Work out the finished part from the listing and answer in its coordinate system (mm). A direction names the side the tool comes from. Coordinates: 2 decimals unless noted, no trailing zeros. Order: outer loops, then holes, each group sorted by start corner. A loop starts at its lowest first (then second) coordinate and runs counter-clockwise, first axis right, second up. Notation, with made-up numbers: M 26,58.25 L 64,58.25 A14 ccw 64,70.25 Z; hole C 37.5,-34 d9. An arc over 180 degrees is marked long. Use a Markdown table: item, result. Add a question column.
from build123d import *

# Parameters (mm, degrees)
SKETCH_R      = 2.5
SKETCH_R_2    = 1.25
PAD_DEPTH     = 3
SKETCH001_R   = 6.5
SKETCH001_R_2 = 4
PAD001_DEPTH  = 10
CHAMFER_SIZE  = 1
SKETCH002_R   = 4
SKETCH002_R_2 = 2.5
PAD002_DEPTH  = 3


with BuildPart() as part:
    # Sketch → Pad (new body)
    with BuildSketch(Plane.XY):
        with BuildLine():
            ThreePointArc((6.928203, 4), (-8, 0), (6.928203, -4))
            Line((10, -4), (6.928203, -4))
            ThreePointArc((10, -4), (14, 0), (10, 4))
            Line((10, 4), (6.928203, 4))
        make_face()
        Circle(SKETCH_R, mode=Mode.SUBTRACT)
        with Locations((10, 0)):
            Circle(SKETCH_R_2, mode=Mode.SUBTRACT)
    extrude(amount=PAD_DEPTH)

    # Sketch001 (on Face8 of Pad) → Pad001 (join)
    with BuildSketch(Plane.XY.offset(3)):
        Circle(SKETCH001_R)
        Circle(SKETCH001_R_2, mode=Mode.SUBTRACT)
    extrude(amount=PAD001_DEPTH)

    # Chamfer
    chamfer_edges = [part.edges().sort_by_distance(p)[0] for p in [
        (-4, 0, 13),
    ]]
    chamfer(chamfer_edges, length=CHAMFER_SIZE)

    # Sketch002 (on Face6 of Chamfer) → Pad002 (join)
    with BuildSketch(Plane.XY.offset(3)):
        Circle(SKETCH002_R)
        Circle(SKETCH002_R_2, mode=Mode.SUBTRACT)
    extrude(amount=PAD002_DEPTH)


solid = part.part
(1) A cutting plane is placed at D-D on x = 5.75. Write down the section's boundary in (y, z), plus the area to 3 significant figures.
(2) Given P1, Ø4, axis at x = 0, y = -1.5, coming from the +Z side; P2, Ø3, axis at x = 10, y = 0, coming from the +Z side; P3, Ø8, axis at x = 3.5, y = -0.5, coming from the +Z side; P4, Ø1.5, axis at x = -5.5, z = 9.5, coming from the -Y side, each flat-ended and moving along its own axis, determine where each tip first touches the part or whether it passes through.
(3) Which of the six approach directions +Z, -Z, +X, -X, +Y, -Y give full straight-line access (tool end or side, diameter ignored) to faces 1 (the cylindrical face through (-0.867, -3.905, 8.958)), 2 (the cylindrical face through (-0.54, -2.44, 2.96)), 3 (the flat face through (8, 4, 1))?
(4) Straight lines are drawn through the part: line 1 (X direction, y = -0.75, z = 2); line 2 (Y direction, x = 0, z = 1.25); line 3 (Y direction, x = 0, z = 9.3). For each, find the intervals that lie inside material, in ascending order.
(5) A cutting plane is placed at C-C on z = 3.75. Write down the section's boundary in (x, y).
(6) A cutting plane is placed at A-A on x = 0. Write down the section's boundary in (y, z).
(7) A cutting plane is placed at B-B on y = 0. Write down the section's boundary in (x, z), plus the area to 4 significant figures.
(8) The mould has two halves that part along X. Classify faces 4 (the cylindrical face through (14, 0, 1)), 5 (the cylindrical face through (-8, 0, 1)), 6 (the cylindrical face through (8.75, 0.05, 1.48)), 7 (the flat face through (8, -4, 1)): pulls with the +X half, pulls with the -X half, needs draft (parallel to the pull), parting line crosses it, or undercut.
From the geometry:
| question | item | result |
|---|---|---|
| 1 | outline | M -5.56,0 L 5.56,0 L 5.56,3 L 3.03,3 L 3.03,13 L -3.03,13 L -3.03,3 L -5.56,3 Z |
| 1 | area | 94.0 mm2 |
| 2 | P1 | stops at z = 6 |
| 2 | P2 | stops at z = 3 |
| 2 | P3 | stops at z = 13 |
| 2 | P4 | stops at y = -4.44 |
| 3 | face 1 | +Z |
| 3 | face 2 | +Z, -Z |
| 3 | face 3 | +Z, -Z, +X, +Y |
| 4 | line 1 | x = -7.96 to -2.38, 2.38 to 9, 11 to 13.93 |
| 4 | line 2 | y = -8 to -2.5, 2.5 to 8 |
| 4 | line 3 | y = -6.5 to -4, 4 to 6.5 |
| 5 | outline | C 0,0 d13; hole C 0,0 d5 |
| 6 | outline | M -8,0 L -2.5,0 L -2.5,6 L -4,6 L -4,12 L -5,13 L -6.5,13 L -6.5,3 L -8,3 Z; M 2.5,0 L 8,0 L 8,3 L 6.5,3 L 6.5,13 L 5,13 L 4,12 L 4,6 L 2.5,6 Z |
| 7 | outline | M -8,0 L -2.5,0 L -2.5,6 L -4,6 L -4,12 L -5,13 L -6.5,13 L -6.5,3 L -8,3 Z; M 2.5,0 L 8.75,0 L 8.75,3 L 6.5,3 L 6.5,13 L 5,13 L 4,12 L 4,6 L 2.5,6 Z; M 11.25,0 L 14,0 L 14,3 L 11.25,3 Z |
| 7 | area | 101.5 mm2 |
| 8 | face 4 | pulls with the +X half |
| 8 | face 5 | parting line crosses it |
| 8 | face 6 | undercut |
| 8 | face 7 | needs draft |
